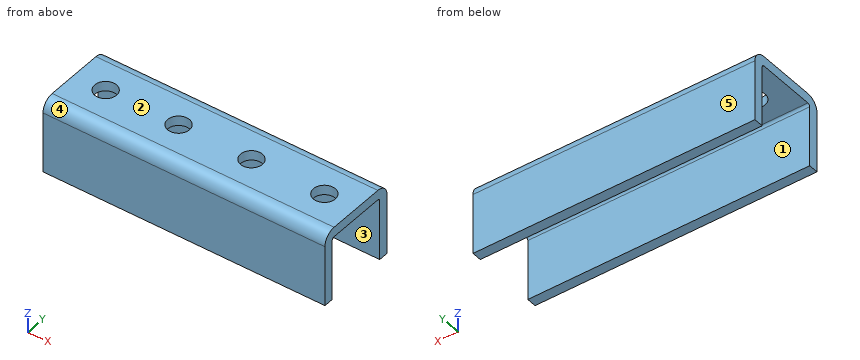
```python
from build123d import *

# Parameters (mm, degrees)
SKETCH1_W           = 184.15
SKETCH1_H           = 53.975
BOSS_EXTRUDE1_DEPTH = 23.8125
FILLET1_R           = 7.9375
SHELL1_T            = -6.35
SKETCH2_R           = 7.14375
CUT_EXTRUDE1_DEPTH  = 47.625


with BuildPart() as part:
    # Sketch1 → Boss-Extrude1 (new, symmetric)
    with BuildSketch(Plane.XY):
        Rectangle(SKETCH1_W, SKETCH1_H)
    extrude(amount=BOSS_EXTRUDE1_DEPTH, both=True)

    # Fillet1
    fillet1_edges = [part.edges().sort_by_distance(p)[0] for p in [
        (0, 26.9875, 23.8125),
        (0, -26.9875, 23.8125),
    ]]
    fillet(fillet1_edges, radius=FILLET1_R)

    # Shell1
    shell1_openings = [part.faces().sort_by_distance(p)[0] for p in [
        (0, 0, -23.8125),
        (92.075, 0, -0.234313972),
        (-92.075, 0, -0.234313972),
    ]]
    offset(amount=SHELL1_T, openings=shell1_openings, kind=Kind.INTERSECTION)

    # Sketch2 → Cut-Extrude1 (cut)
    with BuildSketch(Plane.XY.offset(23.8125)):
        with Locations((-71.4375, 0)):
            Circle(SKETCH2_R)
        with Locations((-23.8125, 0)):
            Circle(SKETCH2_R)
        with Locations((23.8125, 0)):
            Circle(SKETCH2_R)
        with Locations((71.4375, 0)):
            Circle(SKETCH2_R)
    extrude(amount=-CUT_EXTRUDE1_DEPTH, mode=Mode.SUBTRACT)


solid = part.part
```
Could you check a few things on this model? Use its own coordinates, in mm. Face numbers are marked on the shaded views. A direction names the side the tool comes from. Coordinates: 2 decimals unless noted, no trailing zeros. Write each loop counter-clockwise with the first axis right and the second up, starting at its lowest first coordinate (ties: lowest second). Pieces come first, ordered by that corner, then holes. Notation, with made-up numbers: (51, 12) -> (76, 12) arc R30 ccw to (76, 34) -> close; hole circle Ø9 at (19.5, 36). An arc over 180 degrees is marked (long way). Return JSON: item names as keys, results as strings.
(1) I'm going to push flat-ended pins straight in: pin 1 (16.5 mm diameter, centred on x = -23.81, y = 0, fed in from -Z); pin 2 (1 mm diameter, centred on x = -66.5, y = -21, fed in from +Z). Where does each tip first touch, or does it pass through?
Numbers:
{"pin 1": "stops at z = 17.46", "pin 2": "stops at z = 23.68"}
(2) Which directions (+Z, -Z, +X, -X, +Y, -Y) give clear straight access to the entire face, cutting with the end or side of a thin tool? Please do the marked faces 1 and 2.
Numbers:
{"face 1": "-Z, +X, -X", "face 2": "+Z, +X, -X, +Y, -Y"}
(3) Imagine slicing it at A-A, the plane y = 0. Please give me the cut outline in (x, z) (1 decimal).
Numbers:
{"outline": "(-92.1, 17.5) -> (-78.6, 17.5) -> (-78.6, 23.8) -> (-92.1, 23.8) -> close; (-64.3, 17.5) -> (-31, 17.5) -> (-31, 23.8) -> (-64.3, 23.8) -> close; (-16.7, 17.5) -> (16.7, 17.5) -> (16.7, 23.8) -> (-16.7, 23.8) -> close; (31, 17.5) -> (64.3, 17.5) -> (64.3, 23.8) -> (31, 23.8) -> close; (78.6, 17.5) -> (92.1, 17.5) -> (92.1, 23.8) -> (78.6, 23.8) -> close"}
(4) Imagine slicing it at C-C, the plane z = -16.5. Please give me the cut outline in (x, y) (1 decimal).
Numbers:
{"outline": "(-92.1, -27) -> (92.1, -27) -> (92.1, -20.6) -> (-92.1, -20.6) -> close; (-92.1, 20.6) -> (92.1, 20.6) -> (92.1, 27) -> (-92.1, 27) -> close"}
(5) We'd pull the mould along Y, two halves only. Please class the marked faces 3, 4 and 5: +Y half, -Y half, draft (parallel to the pull), parting line (faces both ways), or undercut.
Numbers:
{"face 3": "undercut", "face 4": "-Y half", "face 5": "+Y half"}
(6) I need wall thicknesses on L1, parallel to Y at x = -20, z = -10; L2, parallel to Z at x = -27, y = 17; L3, parallel to Y at x = 62, z = 17. Which ranges of each line are inside material? Lowest first, please.
Numbers:
{"L1": "y = -26.99 to -20.64, 20.64 to 26.99", "L2": "z = 17.46 to 23.81", "L3": "y = -26.91 to -20.17, 20.17 to 26.91"}
